```python
from build123d import *

# Parameters (mm, degrees)
BOSS_EXTRUDE1_DEPTH = 2.286
SKETCH2_R           = 2.159
CUT_EXTRUDE1_DEPTH  = 2.286


with BuildPart() as part:
    # Sketch1 → Boss-Extrude1 (new body)
    with BuildSketch(Plane(origin=(0, 0, 0), x_dir=(1, 0, 0), z_dir=(0, 1, 0))):
        with BuildLine():
            Line((-93.832484615, 46.752607692), (-93.832484615, -17.763392308))
            Line((-93.832484615, -17.763392308), (-90.276484615, -21.319392308))
            Line((-90.276484615, -21.319392308), (-69.956484615, -21.319392308))
            Line((-69.956484615, -21.319392308), (-66.400484615, -17.763392308))
            Line((-66.400484615, -17.763392308), (-66.400484615, 15.002607692))
            ThreePointArc((-66.400484615, 15.002607692), (-63.7966639, 21.288786977), (-57.510484615, 23.892607692))
            Line((-57.510484615, 23.892607692), (-20.680484615, 23.892607692))
            Line((-20.680484615, 23.892607692), (-17.124484615, 27.448607692))
            Line((-17.124484615, 27.448607692), (-17.124484615, 47.768607692))
            Line((-17.124484615, 47.768607692), (-19.664484615, 50.308607692))
            Line((-19.664484615, 50.308607692), (-90.276484615, 50.308607692))
            Line((-90.276484615, 50.308607692), (-93.832484615, 46.752607692))
        make_face()
    extrude(amount=BOSS_EXTRUDE1_DEPTH)

    # Sketch2 → Cut-Extrude1 (cut)
    with BuildSketch(Plane(origin=(0, 2.286, 0), x_dir=(1, 0, 0), z_dir=(0, 1, 0))):
        with Locations((-81.132484615, 37.608607692)):
            Circle(SKETCH2_R)
        with Locations((-81.132484615, 24.908607692)):
            Circle(SKETCH2_R)
        with Locations((-81.132484615, 12.208607692)):
            Circle(SKETCH2_R)
        with Locations((-81.132484615, -0.491392308)):
            Circle(SKETCH2_R)
        with Locations((-81.132484615, -13.191392308)):
            Circle(SKETCH2_R)
        with Locations((-68.432484615, 37.608607692)):
            Circle(SKETCH2_R)
        with Locations((-55.732484615, 37.608607692)):
            Circle(SKETCH2_R)
        with Locations((-43.032484615, 37.608607692)):
            Circle(SKETCH2_R)
        with Locations((-30.332484615, 37.608607692)):
            Circle(SKETCH2_R)
    extrude(amount=-CUT_EXTRUDE1_DEPTH, mode=Mode.SUBTRACT)


solid = part.part
```
Verification items for the finished model (mm, model axes). A direction names the side the tool comes from. Coordinates: 2 decimals unless noted, no trailing zeros. Write each loop counter-clockwise with the first axis right and the second up, starting at its lowest first coordinate (ties: lowest second). Pieces come first, ordered by that corner, then holes. Notation, with made-up numbers: (78.5, -18) - (112.5, -18) arc R28 ccw to (112.5, 19) - close; hole circle Ø1 at (-15, -10). An arc over 180 degrees is marked (long way). One line per question, with ' | ' between items. Start each with the question number.
1. Material ranges on line 1 along Z through (x, y) = (-80, 0.85); line 2 along Z through (x, y) = (-43, 1.85); line 3 along Z through (x, y) = (-48.5, 0.55), recorded low to high.
2. Access from +Z, -Z, +X, -X, +Y, -Y to the whole of each face (thin tool, end or side, straight path). Record for faces 1 (the flat face through (-39, 1, -23.893)), 2 (the cylindrical face through (-44.62, 1.16, -39.07)).
3. Gauge pin test, flat ends, axial feed: P1, Ø2, axis at x = -65, z = -14, coming from the +Y side; P2, Ø1, axis at x = -55.5, y = 1, coming from the +Z side. Record the tip position at first contact, or that the pin passes through.
4. Section check C-C (y = 1.9). Count the separate pieces of the cut face and the enclosed holes in it, plus the area to 3 significant figures.
5. Section check B-B (x = -30). Enter the section's corners in (y, z).
6. Section check A-A (x = -82). Enter the section's corners in (y, z).
7. Section check D-D (z = -4.5). Enter the section's corners in (x, y).
8. Draft check along X on faces 3 (the flat face through (-80, 1, 21.319)), 4 (the flat face through (-17.124, 1, -37)), 5 (the cylindrical face through (-57.32, 1.16, -39.07)). Enter one of: released by +X, released by -X, zero draft, split by the parting line, or undercut.
Computed values:
1) line 1: -50.31 to -39.45, -35.77 to -26.75, -23.07 to -14.05, -10.37 to -1.35, 2.33 to 11.35, 15.03 to 21.32 | line 2: -50.31 to -39.77, -35.45 to -23.89 | line 3: -50.31 to -23.89
2) face 1: +Z, +X, +Y, -Y | face 2: +Y, -Y
3) P1: through | P2: z = -23.89
4) separate pieces: 1 | enclosed holes: 9 | area: 3,120 mm²
5) outline: (0, -50.31) - (2.29, -50.31) - (2.29, -39.74) - (0, -39.74) - close; (0, -35.48) - (2.29, -35.48) - (2.29, -23.89) - (0, -23.89) - close
6) outline: (0, -50.31) - (2.29, -50.31) - (2.29, -39.59) - (0, -39.59) - close; (0, -35.63) - (2.29, -35.63) - (2.29, -26.89) - (0, -26.89) - close; (0, -22.93) - (2.29, -22.93) - (2.29, -14.19) - (0, -14.19) - close; (0, -10.23) - (2.29, -10.23) - (2.29, -1.49) - (0, -1.49) - close; (0, 2.47) - (2.29, 2.47) - (2.29, 11.21) - (0, 11.21) - close; (0, 15.17) - (2.29, 15.17) - (2.29, 21.32) - (0, 21.32) - close
7) outline: (-93.83, 0) - (-66.4, 0) - (-66.4, 2.29) - (-93.83, 2.29) - close
8) face 3: zero draft | face 4: released by +X | face 5: undercut
